Read the model definition and answer for the solid it produces. Units are mm, in the model's axes. A direction names the side the tool comes from. Coordinates: 2 decimals unless noted, no trailing zeros. Write each loop counter-clockwise with the first axis right and the second up, starting at its lowest first coordinate (ties: lowest second). Pieces come first, ordered by that corner, then holes. Notation, with made-up numbers: (33, 31.25) - (76, 31.25) arc R11 cw to (76, 35.25) - close; hole circle Ø9 at (-8.5, -19). An arc over 180 degrees is marked (long way). Use a Markdown table: item, result.
from build123d import *

# Parameters (mm, degrees)
BOSS_EXTRUDE1_DEPTH = 18
SKETCH2_R           = 30
BOSS_EXTRUDE2_DEPTH = 22
SKETCH3_R           = 30
BOSS_EXTRUDE3_DEPTH = 22
SKETCH4_R           = 15
CUT_EXTRUDE1_DEPTH  = 81
CUT_EXTRUDE2_DEPTH  = 45
FILLET1_R           = 7
SKETCH6_R           = 15
BOSS_EXTRUDE4_DEPTH = 45


with BuildPart() as part:
    # Sketch1 → Boss-Extrude1 (new body, symmetric)
    with BuildSketch(Plane.XY):
        with BuildLine():
            Line((31.176914536, 18), (109, 18))
            Line((109, 18), (109, -18))
            Line((109, -18), (31.176914536, -18))
            ThreePointArc((31.176914536, -18), (18, -31.176914536), (0, -36))
            Line((0, -36), (-38, -36))
            Line((-38, -36), (-38, -18))
            Line((-38, -18), (0, -18))
            ThreePointArc((0, -18), (18, 0), (0, 18))
            Line((0, 18), (-38, 18))
            Line((-38, 18), (-38, 36))
            Line((-38, 36), (0, 36))
            ThreePointArc((0, 36), (18, 31.176914536), (31.176914536, 18))
        make_face()
    extrude(amount=BOSS_EXTRUDE1_DEPTH, both=True)

    # Sketch2 → Boss-Extrude2 (add)
    with BuildSketch(Plane.XZ.offset(-18)):
        with Locations((-38, 0)):
            Circle(SKETCH2_R)
    extrude(amount=-BOSS_EXTRUDE2_DEPTH)

    # Sketch3 → Boss-Extrude3 (add)
    with BuildSketch(Plane(origin=(0, -18, 0), x_dir=(1, 0, 0), z_dir=(0, 1, 0))):
        with Locations((-38, 0)):
            Circle(SKETCH3_R)
    extrude(amount=-BOSS_EXTRUDE3_DEPTH)

    # Sketch4 → Cut-Extrude1 (cut, through all)
    with BuildSketch(Plane(origin=(0, 40, 0), x_dir=(1, 0, 0), z_dir=(0, 1, 0))):
        with Locations((-38, 0)):
            Circle(SKETCH4_R)
    extrude(amount=-CUT_EXTRUDE1_DEPTH, mode=Mode.SUBTRACT)

    # Sketch5 → Cut-Extrude2 (cut)
    with BuildSketch(Plane(origin=(109, 0, 0), x_dir=(0, 0, -1), z_dir=(1, 0, 0))):
        Polygon((6, 18), (18, 6), (18, 18), align=None)
        Polygon((18, -18), (18, -6), (6, -18), align=None)
        Polygon((-18, -18), (-6, -18), (-18, -6), align=None)
        Polygon((-18, 18), (-18, 6), (-6, 18), align=None)
    extrude(amount=-CUT_EXTRUDE2_DEPTH, mode=Mode.SUBTRACT)

    # Fillet1
    fillet1_edges = [part.edges().sort_by_distance(p)[0] for p in [
        (64, 12, 12),
        (64, -12, 12),
        (64, -12, -12),
        (64, 12, -12),
    ]]
    fillet(fillet1_edges, radius=FILLET1_R)

    # Sketch6 → Boss-Extrude4 (add)
    with BuildSketch(Plane(origin=(109, 0, 0), x_dir=(0, 0, -1), z_dir=(1, 0, 0))):
        Circle(SKETCH6_R)
    extrude(amount=BOSS_EXTRUDE4_DEPTH)


solid = part.part
(1) A cutting plane is placed at A-A, the plane x = -38. Write down the section's boundary in (y, z), and give its area (3 significant figures).
Report:
| item | result |
|---|---|
| outline | (-40, -30) - (-18, -30) - (-18, -15) - (-40, -15) - close; (-40, 15) - (-18, 15) - (-18, 30) - (-40, 30) - close; (18, -30) - (40, -30) - (40, -15) - (18, -15) - close; (18, 15) - (40, 15) - (40, 30) - (18, 30) - close |
| area | 1,320 mm² |
(2) Each of these flat-tipped pins is pushed along its axis until it touches: P1, Ø0.6, axis at y = -17.5, z = -17, coming from the +X side; P2, Ø3, axis at x = 30.5, z = -16.5, coming from the +Y side; P3, Ø12, axis at x = -36, y = 21.5, coming from the +Z side; P4, Ø7, axis at x = -4, z = 3, coming from the -Y side. Where does it stop, or does it pass through?
Report:
| item | result |
|---|---|
| P1 | stops at x = 64 |
| P2 | stops at y = 21.33 |
| P3 | stops at z = 30 |
| P4 | stops at y = -36 |
(3) A cutting plane is placed at D-D, the plane y = 0. Write down the section's boundary in (x, z).
Report:
| item | result |
|---|---|
| outline | (18, -18) - (109, -18) - (109, -15) - (154, -15) - (154, 15) - (109, 15) - (109, 18) - (18, 18) - close |
(4) A cutting plane is placed at B-B, the plane z = 0. Write down the section's boundary in (x, y), and give its area (3 significant figures).
Report:
| item | result |
|---|---|
| outline | (-68, -40) - (-53, -40) - (-53, -18) - (-68, -18) - close; (-68, 18) - (-53, 18) - (-53, 40) - (-68, 40) - close; (-23, -40) - (-8, -40) - (-8, -36) - (0, -36) arc R36 ccw to (31.18, -18) - (109, -18) - (109, -15) - (154, -15) - (154, 15) - (109, 15) - (109, 18) - (31.18, 18) arc R36 ccw to (0, 36) - (-8, 36) - (-8, 40) - (-23, 40) - (-23, 18) - (0, 18) arc R18 cw to (0, -18) - (-23, -18) - close |
| area | 7,170 mm² |
(5) For faces 1 (the flat face through (90, 12, -12)), 2 (the flat face through (90, -12, 12)), 3 (the flat face through (61, 18, 0)), 4 (the flat face through (90, -12, -12)), 5 (the flat face through (-18, 18, 0)), determine the directions among +Z, -Z, +X, -X, +Y, -Y from which every point of the face is accessible in a straight line to the end or side of a thin tool.
Report:
| item | result |
|---|---|
| face 1 | -Z, +X, +Y |
| face 2 | +Z, +X, -Y |
| face 3 | +Z, -Z, +X, +Y |
| face 4 | -Z, +X, -Y |
| face 5 | +Z, -Z, -X |
(6) A cutting plane is placed at C-C, the plane x = 84.5. Write down the section's boundary in (y, z).
Report:
| item | result |
|---|---|
| outline | (-18, -6) - (-6, -18) - (6, -18) - (18, -6) - (18, 6) - (6, 18) - (-6, 18) - (-18, 6) - close |
(7) The mould has two halves that part along X. Classify faces 6 (the flat face through (90, 12, 12)), 7 (the cylindrical face through (66.922, -13.011, -12.843)), 8 (the cylindrical face through (-52.985, 29.154, -0.66)), 9 (the cylindrical face through (-52.985, -28.846, -0.66)): pulls with the +X half, pulls with the -X half, needs draft (parallel to the pull), parting line crosses it, or undercut.
Report:
| item | result |
|---|---|
| face 6 | needs draft |
| face 7 | pulls with the +X half |
| face 8 | undercut |
| face 9 | undercut |
(8) Straight lines are drawn through the part: L1, parallel to Z at x = -38, y = 23.75; L2, parallel to Y at x = -52, z = -19.5; L3, parallel to X at y = 29, z = 0. For each, find the intervals that lie inside material, in ascending order.
Report:
| item | result |
|---|---|
| L1 | z = -30 to -15, 15 to 30 |
| L2 | y = -40 to -18, 18 to 40 |
| L3 | x = -68 to -53, -23 to 21.33 |
